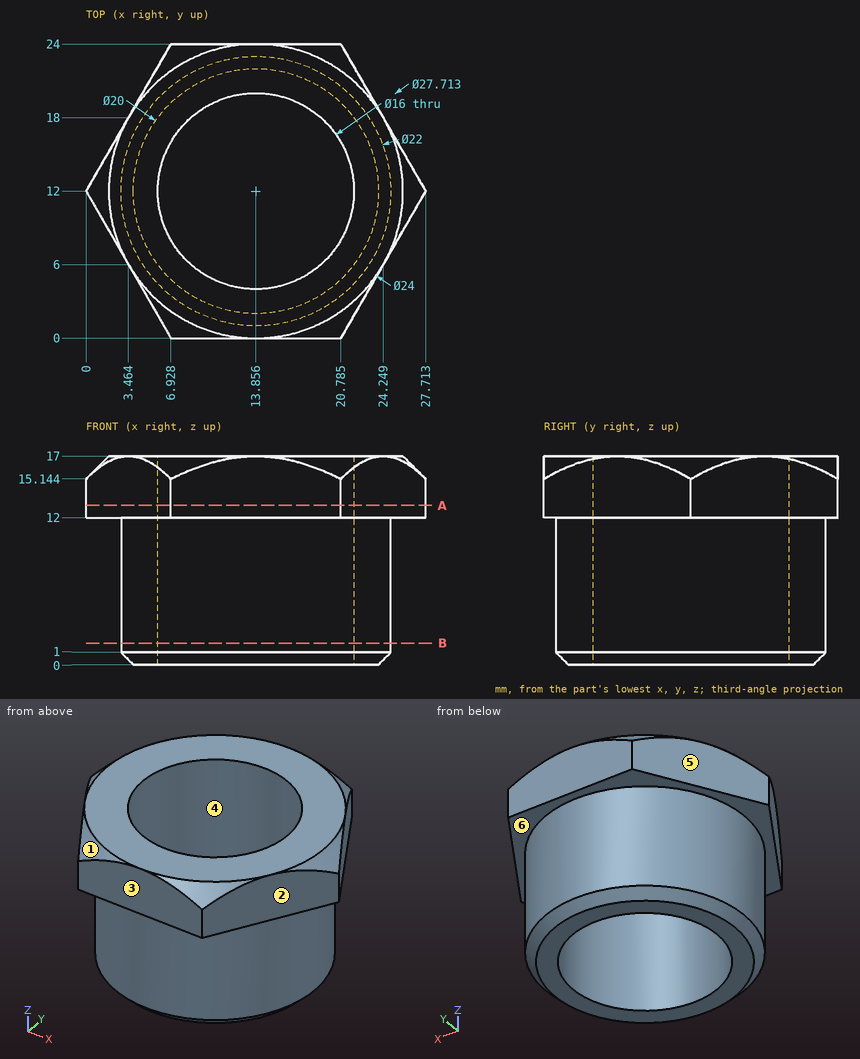
For this review, use the dimensioned drawing (mm, ordinates from the lowest corner) and the shaded views. A direction names the side the tool comes from. Coordinates: 2 decimals unless noted, no trailing zeros. Order: outer loops, then holes, each group sorted by start corner. A loop starts at its lowest first (then second) coordinate and runs counter-clockwise, first axis right, second up. Notation, with made-up numbers: (31.25, 27) -> (44.25, 27) arc R22 ccw to (44.25, 33) -> close; hole circle Ø1 at (81.5, -29.5). An arc over 180 degrees is marked (long way). One line per item, written item: value. Start each with the question number.
Q1. Insertion check: pin 1 Ø3 at (y, z) = (20, 3) entering from -X; pin 2 Ø10 at (y, z) = (5.5, 11.5) entering from +X; pin 3 Ø1 at (y, z) = (13.5, 6.5) entering from +X. Each pin has a flat end and moves straight along its axis. Give the tip position at first contact, or say it passes through.
Q2. Take a section at A-A, the plane z = 13. State the section outline as (x, y) points (1 decimal).
Q3. For probe 1 along Y at (x, z) = (13.75, 13.75); probe 2 along Y at (x, z) = (16.25, 13.5); probe 3 along X at (y, z) = (11.5, 10.75) (1 decimal), list the stretches that pass through material, from the lowest coordinate up.
Q4. Mouldability with a two-part tool opening along X and no side actions: class the marked faces 1, 2, 3 and 4 as pulls with the +X half, pulls with the -X half, needs draft (parallel to the pull), parting line crosses it, or undercut.
Q5. Tool access review of the marked faces 5 and 6: name each direction out of +Z, -Z, +X, -X, +Y, -Y from which nothing blocks a thin tool from reaching the whole face with its end or side.
Q6. Take a section at B-B, the plane z = 1.75. State the section outline as (x, y) points, then the cut area to 3 significant figures.
Values follow:
1. pin 1: stops at x = 4.98
1. pin 2: stops at x = 26.83
1. pin 3: stops at x = 24.81
2. outline: (0, 12) -> (6.9, 0) -> (20.8, 0) -> (27.7, 12) -> (20.8, 24) -> (6.9, 24) -> close; hole circle Ø16 at (13.9, 12)
3. probe 1: y = 0 to 4, 20 to 24
3. probe 2: y = 0 to 4.37, 19.63 to 24
3. probe 3: x = 2.9 to 5.9, 21.8 to 24.8
4. face 1: pulls with the -X half
4. face 2: pulls with the +X half
4. face 3: needs draft
4. face 4: undercut
5. face 5: +Z, -Z, -X, +Y
5. face 6: -Z
6. outline: circle Ø22 at (13.86, 12); hole circle Ø16 at (13.86, 12)
6. area: 179 mm2
